Part model, mm, in its own coordinate system. A direction names the side the tool comes from. Give positions to 0.01 mm unless a question says otherwise; leave off trailing zeros. Order: outer loops, then holes, each group sorted by start corner. A loop starts at its lowest first (then second) coordinate and runs counter-clockwise, first axis right, second up. Notation, with made-up numbers: (27, 80) - (58, 80) arc R15 cw to (58, 85) - close; hole circle Ø3 at (-13.75, 45). An arc over 180 degrees is marked (long way). One line per item, written item: value.
```python
from build123d import *

# Parameters (mm, degrees)
PAD010_DEPTH    = 2.8
FILLET003_R     = 0.4
SKETCH016_R     = 2.5
POCKET003_DEPTH = 2.801


with BuildPart() as part:
    # Sketch010 (on Face2 of ShapeBinder009) → Pad010 (new body)
    with BuildSketch(Plane.XZ.offset(25.388718)):
        with BuildLine():
            Line((42.8, 63.127675), (42.8, 60.327675))
            Line((42.8, 60.327675), (28.8, 60.327675))
            ThreePointArc((28.8, 60.327675), (28.4, 59.927675), (28.8, 59.527675))
            Line((28.8, 59.527675), (42.8, 59.527675))
            Line((42.8, 59.527675), (42.8, 44.127675))
            Line((42.8, 44.127675), (28.8, 44.127675))
            ThreePointArc((28.8, 44.127675), (28.4, 43.727675), (28.8, 43.327675))
            Line((28.8, 43.327675), (42.8, 43.327675))
            Line((42.8, 43.327675), (42.8, 40.527675))
            Line((42.8, 40.527675), (40.8, 39.777675))
            Line((40.8, 40.527675), (40.8, 39.777675))
            Line((40.8, 40.527675), (38, 40.527675))
            Line((38, 40.527675), (38, 38.527675))
            Line((38, 38.527675), (30.535898, 40.527675))
            Line((30.535898, 40.527675), (-30.535898, 40.527675))
            Line((-30.535898, 40.527675), (-38, 38.527675))
            Line((-38, 38.527675), (-38, 40.527675))
            Line((-38, 40.527675), (-40.8, 40.527675))
            Line((-40.8, 40.527675), (-40.8, 39.777675))
            Line((-42.8, 40.527675), (-40.8, 39.777675))
            Line((-42.8, 40.527675), (-42.8, 43.327675))
            Line((-42.8, 43.327675), (-28.8, 43.327675))
            ThreePointArc((-28.8, 43.327675), (-28.4, 43.727675), (-28.8, 44.127675))
            Line((-28.8, 44.127675), (-42.8, 44.127675))
            Line((-42.8, 44.127675), (-42.8, 59.527675))
            Line((-42.8, 59.527675), (-28.8, 59.527675))
            ThreePointArc((-28.8, 59.527675), (-28.4, 59.927675), (-28.8, 60.327675))
            Line((-28.8, 60.327675), (-42.8, 60.327675))
            Line((-42.8, 60.327675), (-42.8, 63.127675))
            Line((-40.8, 63.877675), (-42.8, 63.127675))
            Line((-40.8, 63.127675), (-40.8, 63.877675))
            Line((-40.8, 63.127675), (-38, 63.127675))
            Line((-38, 63.127675), (-38, 65.127675))
            Line((-38, 65.127675), (-30.535898, 63.127675))
            Line((-30.535898, 63.127675), (30.535898, 63.127675))
            Line((30.535898, 63.127675), (38, 65.127675))
            Line((38, 65.127675), (38, 63.127675))
            Line((38, 63.127675), (40.8, 63.127675))
            Line((40.8, 63.127675), (40.8, 63.877675))
            Line((40.8, 63.877675), (42.8, 63.127675))
        make_face()
    extrude(amount=-PAD010_DEPTH)

    # Fillet003
    fillet003_edges = [part.edges().sort_by_distance(p)[0] for p in [
        (-42.8, -23.988718, 60.327675),
        (-42.8, -23.988718, 63.127675),
        (-42.8, -23.988718, 59.527675),
        (-38, -23.988718, 65.127675),
        (38, -23.988718, 65.127675),
        (42.8, -23.988718, 63.127675),
        (42.8, -23.988718, 60.327675),
        (42.8, -23.988718, 59.527675),
        (42.8, -23.988718, 44.127675),
        (42.8, -23.988718, 43.327675),
        (42.8, -23.988718, 40.527675),
        (38, -23.988718, 38.527675),
        (-42.8, -23.988718, 44.127675),
        (-42.8, -23.988718, 43.327675),
        (-42.8, -23.988718, 40.527675),
        (-38, -23.988718, 38.527675),
    ]]
    fillet(fillet003_edges, radius=FILLET003_R)

    # Sketch016 (on Face2 of Fillet003) → Pocket003 (cut, through all)
    with BuildSketch(Plane.XZ.offset(25.388718)):
        with Locations((-25, 51.827675)):
            Circle(SKETCH016_R)
        with Locations((25, 51.827675)):
            Circle(SKETCH016_R)
    extrude(amount=-POCKET003_DEPTH, mode=Mode.SUBTRACT)


solid = part.part
```
1) Which spindle directions (+Z, -Z, +X, -X, +Y, -Y) get a long thin tool onto all of the face, cutting with end or side? Do faces 4 (the face through (-34, -24, 39.6)), 5 (the face through (-36, -24, 59.528)), 6 (the face through (-38, -24, 64)), 7 (the face through (36, -24, 59.528)). Say none if no direction does.
Answer:
face 4: -Z, +Y, -Y
face 5: -X, +Y, -Y
face 6: +Z, +Y, -Y
face 7: +X, +Y, -Y
2) Slice it at D-D on y = -23.95. Count the separate pieces of the cut face and the enclosed holes in it, then the cut area to 3 significant figures.
Answer:
separate pieces: 1
enclosed holes: 2
area: 1,880 mm2
3) Slice it at A-A on x = -25. Write the cut outline in (y, z).
Answer:
outline: (-25.39, 40.53) - (-22.59, 40.53) - (-22.59, 49.33) - (-25.39, 49.33) - close; (-25.39, 54.33) - (-22.59, 54.33) - (-22.59, 63.13) - (-25.39, 63.13) - close
4) Wall check: line 1 along Z through (x, y) = (25, -23.75); line 2 along X through (y, z) = (-25.15, 54); line 3 along Z through (x, y) = (33.5, -22.95). Give the ranges that are in metal, low to high. Write a range as [from, to].
Answer:
line 1: z = [40.53, 49.33], [54.33, 63.13]
line 2: x = [-42.8, -26.24], [-23.76, 23.76], [26.24, 42.8]
line 3: z = [39.73, 43.33], [44.13, 59.53], [60.33, 63.92]
5) Drop flat-ended pins along their axis: P1, Ø3, axis at x = 25, z = 51.83, coming from the +Y side; P2, Ø0.8, axis at x = 40, y = -24.5, coming from the +Z side; P3, Ø1.4, axis at x = -39, y = -24, coming from the -Z side; P4, Ø1.4, axis at x = -32.5, y = -24, coming from the -Z side. Give the stop position or say it passes through.
Answer:
P1: passes through
P2: stops at z = 63.13
P3: stops at z = 40.53
P4: stops at z = 39.81
6) Two-plate mould, pull along Z, no slides. Class faces 1 (the face through (41.658, -24.008, 63.556)), 2 (the face through (36, -24, 43.328)), 3 (the face through (42.8, -24, 62)): pulls with the +Z half, pulls with the -Z half, needs draft (parallel to the pull), parting line crosses it, or undercut.
Answer:
face 1: pulls with the +Z half
face 2: undercut
face 3: needs draft
7) Slice it at C-C on x = 6.5. Write the cut outline in (y, z).
Answer:
outline: (-25.39, 40.53) - (-22.59, 40.53) - (-22.59, 63.13) - (-25.39, 63.13) - close
8) Slice it at B-B on x = 33. Write the cut outline in (y, z).
Answer:
outline: (-25.39, 39.87) - (-22.59, 39.87) - (-22.59, 43.33) - (-25.39, 43.33) - close; (-25.39, 44.13) - (-22.59, 44.13) - (-22.59, 59.53) - (-25.39, 59.53) - close; (-25.39, 60.33) - (-22.59, 60.33) - (-22.59, 63.79) - (-25.39, 63.79) - close
